The listing builds one solid part. Answer for the finished solid, in the listing's coordinates (mm). Face numbers are marked on the shaded views. A direction names the side the tool comes from. Give positions to 0.01 mm unless a question says otherwise; leave off trailing zeros. Write each loop counter-clockwise with the first axis right and the second up, starting at its lowest first coordinate (ties: lowest second). Pieces come first, ordered by that corner, then holes. Notation, with made-up numbers: (50, -1.5) - (107, -1.5) arc R17 cw to (107, 21.5) - close; hole circle Ø1 at (55.5, -15.75). An arc over 180 degrees is marked (long way). One line per question, with ' | ' between items. Start each with the question number.
1. For the marked faces 4, 5, 6 and 7, determine the directions among +Z, -Z, +X, -X, +Y, -Y from which every point of the face is accessible in a straight line to the end or side of a thin tool.
2. The mould has two halves that part along X. Classify the marked faces 1, 2 and 3: +X half, -X half, draft (parallel to the pull), parting line (faces both ways), or undercut.
3. A cutting plane is placed at A-A (y = 24). Determine the outline of the cut face in (x, z).
4. Given P1, Ø12, axis at x = -5, y = 67, coming from the -Z side; P2, Ø5, axis at x = 4, z = 22, coming from the +Y side; P3, Ø3, axis at x = 5.5, z = 27, coming from the +Y side, each flat-ended and moving along its own axis, determine where each tip first touches the part or whether it passes through.
5. Find the intervals of material crossed by L1, parallel to Z at x = 0, y = 62; L2, parallel to X at y = 15, z = 27, in increasing order. Write a range as from..to.
6. A cutting plane is placed at D-D (x = 21). Determine the outline of the cut face in (y, z), then the cut area to 3 significant figures.
7. A cutting plane is placed at C-C (z = -18). Determine the outline of the cut face in (x, y).
8. A cutting plane is placed at B-B (y = 51.5). Determine the outline of the cut face in (x, z), then the cut area to 3 significant figures.
```python
from build123d import *

# Parameters (mm, degrees)
ESQUISSE1_W             = 54.5
ESQUISSE1_H             = 54.5
BOSS_EXTRU_1_DEPTH      = 100
ENL_V_MAT_EXTRU_1_DEPTH = 55.5
ESQUISSE4_W             = 44.5
ESQUISSE4_H             = 44.5
ENL_V_MAT_EXTRU_3_DEPTH = 101
ENL_V_MAT_EXTRU_7_DEPTH = 55.5
BOSS_EXTRU_2_DEPTH      = 5


with BuildPart() as part:
    # Esquisse1 → Boss.-Extru.1 (new body)
    with BuildSketch(Plane(origin=(0, 0, 0), x_dir=(1, 0, 0), z_dir=(0, 1, 0))):
        Rectangle(ESQUISSE1_W, ESQUISSE1_H)
    extrude(amount=BOSS_EXTRU_1_DEPTH)

    # Esquisse2 → Enlèv. mat.-Extru.1 (cut, through all)
    with BuildSketch(Plane(origin=(27.25, 0, 0), x_dir=(0, 0, -1), z_dir=(1, 0, 0))):
        Polygon((-22.25, 0), (22.25, 0), (22.25, 44.5), (22.25, 57.346043489), (0, 70.192086979), (-22.25, 57.346043489), (-22.25, 44.5), align=None)
    extrude(amount=-ENL_V_MAT_EXTRU_1_DEPTH, mode=Mode.SUBTRACT)

    # Esquisse4 → Enlèv. mat.-Extru.3 (cut, through all)
    with BuildSketch(Plane(origin=(0, 100, 0), x_dir=(1, 0, 0), z_dir=(0, 1, 0))):
        Rectangle(ESQUISSE4_W, ESQUISSE4_H)
    extrude(amount=-ENL_V_MAT_EXTRU_3_DEPTH, mode=Mode.SUBTRACT)

    # Esquisse6 → Enlèv. mat.-Extru.7 (cut, through all)
    with BuildSketch(Plane(origin=(0, 0, -27.25), x_dir=(-1, 0, 0), z_dir=(0, 0, -1))):
        Polygon((0, 109.959292144), (-17.25, 100), (-17.25, 80.081415713), (0, 70.122123569), (17.25, 80.081415713), (17.25, 100), align=None)
        with BuildLine():
            Line((17.25, 0), (-17.25, 0))
            Line((-17.25, 0), (-17.25, 32.75))
            ThreePointArc((-17.25, 32.75), (0, 50), (17.25, 32.75))
            Line((17.25, 32.75), (17.25, 0))
        make_face()
    extrude(amount=-ENL_V_MAT_EXTRU_7_DEPTH, mode=Mode.SUBTRACT)

    # Esquisse11 → Boss.-Extru.2 (add)
    with BuildSketch(Plane(origin=(0, 0, 0), x_dir=(1, 0, 0), z_dir=(0, 1, 0))):
        with BuildLine():
            Line((19.25, 37.25), (19.25, 32.25))
            ThreePointArc((19.25, 32.25), (22.25, 29.25), (25.25, 32.25))
            Line((25.25, 32.25), (25.25, 37.25))
            Line((25.25, 37.25), (27.25, 37.25))
            Line((27.25, 37.25), (27.25, 22.25))
            Line((27.25, 22.25), (17.25, 22.25))
            Line((17.25, 22.25), (17.25, 37.25))
            Line((17.25, 37.25), (19.25, 37.25))
        make_face()
        with BuildLine():
            Line((-17.25, 22.25), (-27.25, 22.25))
            Line((-27.25, 22.25), (-27.25, 37.25))
            Line((-27.25, 37.25), (-25.25, 37.25))
            Line((-25.25, 37.25), (-25.25, 32.25))
            ThreePointArc((-25.25, 32.25), (-22.25, 29.25), (-19.25, 32.25))
            Line((-19.25, 32.25), (-19.25, 37.25))
            Line((-19.25, 37.25), (-17.25, 37.25))
            Line((-17.25, 37.25), (-17.25, 22.25))
        make_face()
        with BuildLine():
            Line((17.25, -22.25), (27.25, -22.25))
            Line((27.25, -22.25), (27.25, -37.25))
            Line((27.25, -37.25), (25.25, -37.25))
            Line((25.25, -37.25), (25.25, -32.25))
            ThreePointArc((25.25, -32.25), (22.25, -29.25), (19.25, -32.25))
            Line((19.25, -32.25), (19.25, -37.25))
            Line((19.25, -37.25), (17.25, -37.25))
            Line((17.25, -37.25), (17.25, -22.25))
        make_face()
        with BuildLine():
            Line((-19.25, -37.25), (-19.25, -32.25))
            ThreePointArc((-19.25, -32.25), (-22.25, -29.25), (-25.25, -32.25))
            Line((-25.25, -32.25), (-25.25, -37.25))
            Line((-25.25, -37.25), (-27.25, -37.25))
            Line((-27.25, -37.25), (-27.25, -22.25))
            Line((-27.25, -22.25), (-17.25, -22.25))
            Line((-17.25, -22.25), (-17.25, -37.25))
            Line((-17.25, -37.25), (-19.25, -37.25))
        make_face()
    extrude(amount=BOSS_EXTRU_2_DEPTH)


solid = part.part
```
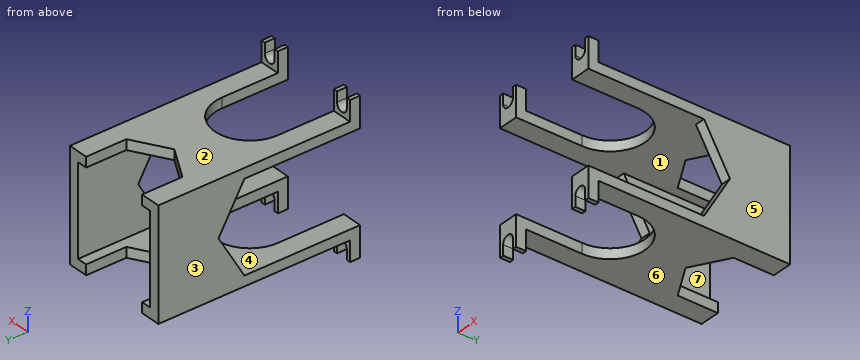
Determined:
1) face 4: -Y | face 5: +Z, -Z, +X, +Y, -Y | face 6: -Z, +X, -X, +Y | face 7: +Y, -Y
2) face 1: undercut | face 2: draft | face 3: -X half
3) outline: (-27.25, -27.25) - (-17.25, -27.25) - (-17.25, -22.25) - (-27.25, -22.25) - close; (-27.25, 22.25) - (-17.25, 22.25) - (-17.25, 27.25) - (-27.25, 27.25) - close; (17.25, -27.25) - (27.25, -27.25) - (27.25, -22.25) - (17.25, -22.25) - close; (17.25, 22.25) - (27.25, 22.25) - (27.25, 27.25) - (17.25, 27.25) - close
4) P1: z = -27.25 | P2: y = 73.87 | P3: y = 74.16
5) L1: -27.25..-22.25, 22.25..27.25 | L2: -27.25..-17.25, 17.25..27.25
6) outline: (0, -29.52) - (5, -29.52) - (5, -27.25) - (100, -27.25) - (100, -22.25) - (0, -22.25) - close; (0, 22.25) - (100, 22.25) - (100, 27.25) - (5, 27.25) - (5, 29.52) - (0, 29.52) - close | area: 1,020 mm2
7) outline: (-27.25, 59.8) - (-22.25, 59.8) - (-22.25, 100) - (-27.25, 100) - close; (22.25, 59.8) - (27.25, 59.8) - (27.25, 100) - (22.25, 100) - close
8) outline: (-27.25, -27.25) - (27.25, -27.25) - (27.25, -22.25) - (-27.25, -22.25) - close; (-27.25, 22.25) - (27.25, 22.25) - (27.25, 27.25) - (-27.25, 27.25) - close | area: 545 mm2
